```python
from build123d import *

# Parameters (mm, degrees)
CUT_EXTRUDE2_DEPTH  = 2
SKETCH4_R           = 1.5
CUT_EXTRUDE3_DEPTH  = 30.819624498
CUT_EXTRUDE4_DEPTH  = 27.804663864
CUT_EXTRUDE5_START  = -10
SKETCH6_R           = 8
SKETCH6_R_2         = 6
CUT_EXTRUDE5_DEPTH  = 10
CUT_EXTRUDE6_DEPTH  = 30.346379825
BOSS_EXTRUDE1_DEPTH = 4
SKETCH9_R           = 1
CUT_EXTRUDE7_DEPTH  = 30.012178231
FILLET1_R           = 2


with BuildPart() as part:
    # Sketch2 → Revolve1 (revolve)
    with BuildSketch(Plane.XY, mode=Mode.PRIVATE) as revolve1_sk:
        Polygon((0, 26.1), (-6, 26.1), (-6, 17.1), (-5.75, 17.1), (-5.75, 16), (-6, 16), (-6, 4), (-8, 4), (-8, 0), (-7, 0), (-7, 1.8), (0, 1.8), align=None)
    revolve(revolve1_sk.sketch.rotate(Axis((0, 0, 0), (0, 1, 0)), 270), axis=Axis((0, 0, 0), (0, 1, 0)))

    # Sketch3 → Cut-Extrude2 (cut)
    with BuildSketch(Plane.ZY.offset(6)):
        with BuildLine():
            Line((9, 26.1), (-9, 26.1))
            ThreePointArc((-9, 26.1), (-6.171572875, 24.928427125), (-5, 22.1))
            ThreePointArc((-5, 22.1), (-3.828427125, 19.271572875), (-1, 18.1))
            Line((-1, 18.1), (1, 18.1))
            ThreePointArc((1, 18.1), (3.828427125, 19.271572875), (5, 22.1))
            ThreePointArc((5, 22.1), (6.171572875, 24.928427125), (9, 26.1))
        make_face()
    cut_extrude2 = extrude(amount=-CUT_EXTRUDE2_DEPTH, mode=Mode.SUBTRACT)

    # Mirror1: Cut-Extrude2 across plane
    add(cut_extrude2.mirror(Plane(origin=(0, 0, 0), x_dir=(0, 0, 1), z_dir=(1, 0, 0))), mode=Mode.SUBTRACT)

    # Sketch4 → Cut-Extrude3 (cut, through all)
    with BuildSketch(Plane.ZY.offset(4)):
        with Locations((0, 21.1)):
            Circle(SKETCH4_R)
    extrude(amount=-CUT_EXTRUDE3_DEPTH, mode=Mode.SUBTRACT)

    # Sketch5 → Cut-Extrude4 (cut, through all)
    with BuildSketch(Plane.XZ.offset(-1.8)):
        with BuildLine():
            Line((2.291287847, 1), (-2.291287847, 1))
            ThreePointArc((-2.291287847, 1), (-0.510774109, -2.447265782), (2.5, 0))
            ThreePointArc((2.5, 0), (2.447265782, 0.510774109), (2.291287847, 1))
        make_face()
    extrude(amount=-CUT_EXTRUDE4_DEPTH, mode=Mode.SUBTRACT)

    # Sketch6 → Cut-Extrude5 (cut)
    with BuildSketch(Plane(origin=(0, 4, 0), x_dir=(1, 0, 0), z_dir=(0, 1, 0)).offset(CUT_EXTRUDE5_START)):
        Circle(SKETCH6_R)
        with Locations(Location((0, 0, 0), (0, 0, 90))):
            Circle(SKETCH6_R_2, mode=Mode.SUBTRACT)
    extrude(amount=CUT_EXTRUDE5_DEPTH, mode=Mode.SUBTRACT)

    # Sketch7 → Cut-Extrude6 (cut, through all)
    with BuildSketch(Plane(origin=(6, 0, 0), x_dir=(0, 0, -1), z_dir=(1, 0, 0))):
        with BuildLine():
            Line((-1, 1.8), (-1, 6.8))
            ThreePointArc((-1, 6.8), (0, 7.8), (1, 6.8))
            Line((1, 6.8), (1, 1.8))
            Line((1, 1.8), (-1, 1.8))
        make_face()
    extrude(amount=-CUT_EXTRUDE6_DEPTH, mode=Mode.SUBTRACT)

    # Sketch8 → Boss-Extrude1 (add)
    with BuildSketch(Plane.XZ.offset(-1.8)):
        with BuildLine():
            Line((-8.916079783, -3), (-5.196152423, -3))
            ThreePointArc((-5.196152423, -3), (-5.645389814, -2.032135293), (-5.916079783, -1))
            Line((-5.916079783, -1), (-8.916079783, -1))
            Line((-8.916079783, -1), (-8.916079783, -3))
        make_face()
        with BuildLine():
            ThreePointArc((-5.916079783, 1), (-5.645389814, 2.032135293), (-5.196152423, 3))
            Line((-5.196152423, 3), (-8.916079783, 3))
            Line((-8.916079783, 3), (-8.916079783, 1))
            Line((-8.916079783, 1), (-5.916079783, 1))
        make_face()
        with BuildLine():
            ThreePointArc((5.196152423, 3), (5.645389814, 2.032135293), (5.916079783, 1))
            Line((5.916079783, 1), (8.916079783, 1))
            Line((8.916079783, 1), (8.916079783, 3))
            Line((8.916079783, 3), (5.196152423, 3))
        make_face()
        with BuildLine():
            ThreePointArc((5.196152423, -3), (5.645389814, -2.032135293), (5.916079783, -1))
            Line((5.916079783, -1), (8.916079783, -1))
            Line((8.916079783, -1), (8.916079783, -3))
            Line((8.916079783, -3), (5.196152423, -3))
        make_face()
    extrude(amount=-BOSS_EXTRUDE1_DEPTH)

    # Sketch9 → Cut-Extrude7 (cut, through all)
    with BuildSketch(Plane(origin=(0, 0, -3), x_dir=(-1, 0, 0), z_dir=(0, 0, -1))):
        with Locations((-6.916079783, 3.8)):
            Circle(SKETCH9_R)
        with Locations((6.916079783, 3.8)):
            Circle(SKETCH9_R)
    extrude(amount=-CUT_EXTRUDE7_DEPTH, mode=Mode.SUBTRACT)

    # Fillet1
    fillet1_edges = [part.edges().sort_by_distance(p)[0] for p in [
        (-8.916079783, 5.8, 2),
        (-8.916079783, 1.8, 2),
        (-8.916079783, 1.8, -2),
        (-8.916079783, 5.8, -2),
        (8.916079783, 1.8, 2),
        (8.916079783, 5.8, 2),
        (8.916079783, 1.8, -2),
        (8.916079783, 5.8, -2),
    ]]
    fillet(fillet1_edges, radius=FILLET1_R - 0.0001)  # a hair under: the kernel refuses the full size


solid = part.part
```
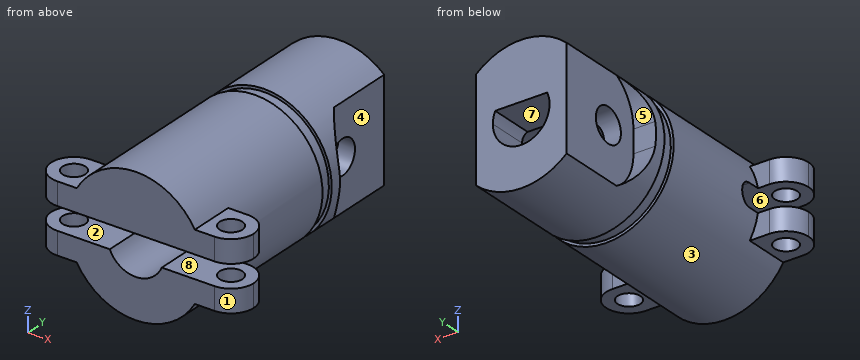
Geometry check sheet. Reference: the model listing, model coordinates, mm. Face numbers are marked on the shaded views. A direction names the side the tool comes from. Give positions to 0.01 mm unless a question says otherwise; leave off trailing zeros. Write each loop counter-clockwise with the first axis right and the second up, starting at its lowest first coordinate (ties: lowest second). Pieces come first, ordered by that corner, then holes. Notation, with made-up numbers: (42, 70.25) - (87, 70.25) arc R24 cw to (87, 95.25) - close; hole circle Ø1 at (74.5, 80.5). An arc over 180 degrees is marked (long way). Use a Markdown table: item, result.
Q1. Section check D-D, the plane y = 8.25. Enter the section's corners in (x, z).
Computed:
| item | result |
|---|---|
| outline | circle Ø12 at (0, 0); hole (-2.29, 1) arc R2.5 ccw (long way) to (2.29, 1) - close |
Q2. Section check A-A, the plane y = 21.1. Enter the section's corners in (x, z), then the cut area to 3 significant figures.
Computed:
| item | result |
|---|---|
| outline | (-4, -4.47) arc R6 ccw to (4, -4.47) - (4, -1.5) - (2, -1.5) arc R2.5 cw to (-2, -1.5) - (-4, -1.5) - close; (-4, 1.5) - (4, 1.5) - (4, 4.47) arc R6 ccw to (-4, 4.47) - close |
| area | 61.5 mm² |
Q3. Set-up check for the marked faces 4, 5, 6, 7 and 8: record each of +Z, -Z, +X, -X, +Y, -Y from which the full face is reachable in a straight line by a thin tool's end or side.
Computed:
| item | result |
|---|---|
| face 4 | +X, +Y |
| face 5 | -X, +Y |
| face 6 | -Y |
| face 7 | +Y, -Y |
| face 8 | +X, -X, -Y |
Q4. Section check C-C, the plane z = -2. Give the number of separate pieces and of enclosed holes in the cut face, then the cut area to 3 significant figures.
Computed:
| item | result |
|---|---|
| separate pieces | 2 |
| enclosed holes | 2 |
| area | 192 mm² |
Q5. Go/stop test with flat-tipped pins: P1, Ø2.5, axis at x = 6.92, y = 3.8, coming from the +Z side; P2, Ø4, axis at y = 15.5, z = 3, coming from the -X side; P3, Ø0.5, axis at x = 6, z = 2, coming from the +Y side. Record where each tip stops, or that it passes through.
Computed:
| item | result |
|---|---|
| P1 | stops at z = 3 |
| P2 | stops at x = -5.92 |
| P3 | stops at y = 5.8 |
Q6. Draft check along Z on the marked faces 1, 2 and 3. Enter one of: pulls with the +Z half, pulls with the -Z half, needs draft (parallel to the pull), parting line crosses it, or undercut.
Computed:
| item | result |
|---|---|
| face 1 | needs draft |
| face 2 | undercut |
| face 3 | parting line crosses it |
Q7. Thickness scan on L1, parallel to X at y = 17.75, z = -2; L2, parallel to X at y = 23.5, z = -3; L3, parallel to X at y = 25, z = 0.5. Record the ranges inside material, lowest first. Write a range as [from, to].
Computed:
| item | result |
|---|---|
| L1 | x = [-5.66, -1.5], [1.5, 5.66] |
| L2 | x = [-4, 4] |
| L3 | x = [-4, -2.45], [2.45, 4] |
Q8. Section check B-B, the plane x = 0. Enter the section's corners in (y, z).
Computed:
| item | result |
|---|---|
| outline | (1.8, -6) - (16, -6) - (16, -5.75) - (17.1, -5.75) - (17.1, -6) - (26.1, -6) - (26.1, -2.5) - (1.8, -2.5) - close; (1.8, 1) - (19.98, 1) arc R1.5 cw to (22.22, 1) - (26.1, 1) - (26.1, 6) - (17.1, 6) - (17.1, 5.75) - (16, 5.75) - (16, 6) - (1.8, 6) - close |
